```python
from build123d import *

# Parameters (mm, degrees)
SALIENTE_EXTRUIR1_DEPTH = 220
CORTAR_EXTRUIR2_DEPTH   = 14
CROQUIS2_9_W            = 24
CROQUIS2_9_H            = 1
CROQUIS2_9_W_2          = 5
CORTAR_EXTRUIR3_DEPTH   = 3
CROQUIS4_R              = 1.5
CORTAR_EXTRUIR4_DEPTH   = 10
CROQUIS5_R              = 2
CORTAR_EXTRUIR5_DEPTH   = 36
CROQUIS6_W              = 55
CROQUIS6_H              = 15
CORTAR_EXTRUIR7_DEPTH   = 10
CORTAR_EXTRUIR8_DEPTH   = 30


with BuildPart() as part:
    # Croquis1 → Saliente-Extruir1 (new body)
    with BuildSketch(Plane.XY):
        with BuildLine():
            Line((0, 37), (0, 8.15))
            ThreePointArc((0, 8.15), (-8.15, 0), (0, -8.15))
            Line((0, -8.15), (0, -37))
            Line((0, -37), (-33, -37))
            ThreePointArc((-33, -37), (-34.414213562, -36.414213562), (-35, -35))
            Line((-35, -35), (-35, 35))
            ThreePointArc((-35, 35), (-34.414213562, 36.414213562), (-33, 37))
            Line((-33, 37), (0, 37))
        make_face()
    extrude(amount=SALIENTE_EXTRUIR1_DEPTH)

    # Croquis2 → Cortar-Extruir2 (cut)
    with BuildSketch(Plane.ZY.offset(35)):
        Polygon((50.34, -1.15), (82.34, -1.15), (82.34, -17.5), (156.34, -17.5), (156.34, -1.15), (169.34, -1.15), (169.34, -13.5), (196.34, -13.5), (196.34, 13.5), (169.34, 13.5), (169.34, 1.15), (156.34, 1.15), (156.34, 17.5), (82.34, 17.5), (82.34, 1.15), (50.34, 1.15), (50.34, 10.5), (10, 10.5), (10, -10.5), (50.34, -10.5), align=None)
    extrude(amount=-CORTAR_EXTRUIR2_DEPTH, mode=Mode.SUBTRACT)

    # Croquis2_9 → Cortar-Extruir3 (cut)
    with BuildSketch(Plane.ZY.offset(35)):
        Polygon((54.34, 1.15), (54.34, 2.15), (54.34, 14.5), (6, 14.5), (6, -14.5), (54.34, -14.5), (54.34, -2.15), (54.34, -1.15), (50.34, -1.15), (50.34, -10.5), (10, -10.5), (10, 10.5), (50.34, 10.5), (50.34, 1.15), align=None)
        with Locations((66.34, 1.65)):
            Rectangle(CROQUIS2_9_W, CROQUIS2_9_H)
        with Locations((66.34, -1.65)):
            Rectangle(CROQUIS2_9_W, CROQUIS2_9_H)
        Polygon((78.34, 21.5), (78.34, 2.15), (78.34, 1.15), (82.34, 1.15), (82.34, 17.5), (156.34, 17.5), (156.34, 1.15), (160.34, 1.15), (160.34, 2.15), (160.34, 21.5), align=None)
        Polygon((82.34, -1.15), (78.34, -1.15), (78.34, -2.15), (78.34, -21.5), (160.34, -21.5), (160.34, -2.15), (160.34, -1.15), (156.34, -1.15), (156.34, -17.5), (82.34, -17.5), align=None)
        with Locations((162.84, 1.65)):
            Rectangle(CROQUIS2_9_W_2, CROQUIS2_9_H)
        with Locations((162.84, -1.65)):
            Rectangle(CROQUIS2_9_W_2, CROQUIS2_9_H)
        Polygon((165.34, 17.5), (165.34, 2.15), (165.34, 1.15), (169.34, 1.15), (169.34, 13.5), (196.34, 13.5), (196.34, -13.5), (169.34, -13.5), (169.34, -1.15), (165.34, -1.15), (165.34, -2.15), (165.34, -17.5), (200.34, -17.5), (200.34, 17.5), align=None)
    extrude(amount=-CORTAR_EXTRUIR3_DEPTH, mode=Mode.SUBTRACT)

    # Croquis4 → Cortar-Extruir4 (cut)
    with BuildSketch(Plane.ZY.offset(35)):
        with Locations((8, 12.5)):
            Circle(CROQUIS4_R)
        with Locations((8, -12.5)):
            Circle(CROQUIS4_R)
        with Locations((52.34, 12.5)):
            Circle(CROQUIS4_R)
        with Locations((52.34, -12.5)):
            Circle(CROQUIS4_R)
        with Locations((80.34, 19.5)):
            Circle(CROQUIS4_R)
        with Locations((158.34, 19.5)):
            Circle(CROQUIS4_R)
        with Locations((80.34, -19.5)):
            Circle(CROQUIS4_R)
        with Locations((158.34, -19.5)):
            Circle(CROQUIS4_R)
        with Locations((167.34, 15.5)):
            Circle(CROQUIS4_R)
        with Locations((198.34, 15.5)):
            Circle(CROQUIS4_R)
        with Locations((167.34, -15.5)):
            Circle(CROQUIS4_R)
        with Locations((198.34, -15.5)):
            Circle(CROQUIS4_R)
    extrude(amount=-CORTAR_EXTRUIR4_DEPTH, mode=Mode.SUBTRACT)

    # Croquis5 → Cortar-Extruir5 (cut, through all)
    with BuildSketch(Plane.ZY.offset(35)):
        with Locations((40, 31.5)):
            Circle(CROQUIS5_R)
        with Locations((40, -31.5)):
            Circle(CROQUIS5_R)
        with Locations((180, 31.5)):
            Circle(CROQUIS5_R)
        with Locations((180, -31.5)):
            Circle(CROQUIS5_R)
    extrude(amount=-CORTAR_EXTRUIR5_DEPTH, mode=Mode.SUBTRACT)

    # Croquis6 → Cortar-Extruir7 (cut)
    with BuildSketch(Plane.ZY.offset(21)):
        with Locations((128.84, 10)):
            Rectangle(CROQUIS6_W, CROQUIS6_H)
    extrude(amount=-CORTAR_EXTRUIR7_DEPTH, mode=Mode.SUBTRACT)

    # Croquis12 → Cortar-Extruir8 (cut)
    with BuildSketch(Plane(origin=(0, 37, 0), x_dir=(1, 0, 0), z_dir=(0, 1, 0))):
        Polygon((-19.700712137, -82.34), (-18.7, -82.34), (-18.7, -106.34), (-28.2, -106.34), (-28.2, -82.34), align=None)
    extrude(amount=-CORTAR_EXTRUIR8_DEPTH, mode=Mode.SUBTRACT)


solid = part.part
```
Read the model definition and answer for the solid it produces. Units are mm, in the model's axes. A direction names the side the tool comes from. Coordinates: 2 decimals unless noted, no trailing zeros. Order: outer loops, then holes, each group sorted by start corner. A loop starts at its lowest first (then second) coordinate and runs counter-clockwise, first axis right, second up. Notation, with made-up numbers: (-20, -28.5) - (-6, -28.5) arc R16 ccw to (-6, -21.5) - close; hole circle Ø9 at (76.25, 15.25). An arc over 180 degrees is marked (long way). Answer as a JSON object with one key per item and string values. Group by question number.
Item 1: Flat-ended cylindrical pins translate along their axes: P1, Ø10, axis at y = 12, z = 140.5, coming from the -X side; P2, Ø2, axis at y = 16, z = 79.5, coming from the -X side; P3, Ø3, axis at y = 2, z = 25.5, coming from the -X side; P4, Ø3, axis at y = 31.5, z = 180, coming from the +X side. Find the tip coordinate at first contact, or state that the pin passes through.
Item 2: Consider probe 1 along Y at (x, z) = (-17.5, 40); probe 2 along Y at (x, z) = (-28.5, 80.34); probe 3 along X at (y, z) = (18, 89). Determine where each line is inside the solid, lowest interval first. Write a range as from..to.
Item 3: Section D-D (z = 203.5) is taken. Give the vertices of the cut face in (x, y), plus the area to 3 significant figures.
Item 4: Section B-B (x = -6) is taken. Give the vertices of the cut face in (y, z), plus the area to 3 significant figures.
Item 5: A tool of negligible diameter and unlimited length cuts with its end or side. For faces 1 (the face through (-22, 17.5, 128)), 2 (the face through (-23, 27, 106.34)), 3 (the face through (-17, 1, 0)), from which of +Z, -Z, +X, -X, +Y, -Y can it reach the whole face along a straight path? Write none if from no direction.
Item 6: The mould has two halves that part along Y. Classify faces 4 (the face through (-16, -37, 108)), 5 (the face through (-18.7, 22, 94)), 6 (the face through (-17, 37, 108)), 7 (the face through (-27, -1.15, 163)): +Y half, -Y half, draft (parallel to the pull), parting line (faces both ways), or undercut.
Item 7: Section A-A (y = 23.5) is taken. Give the vertices of the cut face in (x, z), plus the area to 3 significant figures.
Item 8: Section C-C (z = 40) is taken. Give the vertices of the cut face in (x, y), plus the area to 3 significant figures.
Results are:
{
 "1": {"P1": "stops at x = -11", "P2": "stops at x = -32", "P3": "stops at x = -21", "P4": "passes through"},
 "2": {"probe 1": "y = -37..-33.5, -29.5..29.5, 33.5..37", "probe 2": "y = -37..-21, -18..-1.15, 1.15..18, 21..37", "probe 3": "x = -32..-28.2, -18.7..0"},
 "3": {"outline": "(-35, -35) arc R2 ccw to (-33, -37) - (0, -37) - (0, -8.15) arc R8.15 cw to (0, 8.15) - (0, 37) - (-33, 37) arc R2 ccw to (-35, 35) - close", "area": "2,480 mm^2"},
 "4": {"outline": "(-37, 0) - (-5.52, 0) - (-5.52, 220) - (-37, 220) - close; (5.52, 0) - (37, 0) - (37, 220) - (5.52, 220) - close; hole circle Ø4 at (-31.5, 40); hole circle Ø4 at (-31.5, 180); hole circle Ø4 at (31.5, 40); hole circle Ø4 at (31.5, 180)", "area": "13,800 mm^2"},
 "5": {"face 1": "-X", "face 2": "+Y", "face 3": "-Z, +X, -X, +Y, -Y"},
 "6": {"face 4": "-Y half", "face 5": "draft", "face 6": "+Y half", "face 7": "undercut"},
 "7": {"outline": "(-35, 0) - (0, 0) - (0, 220) - (-35, 220) - close; hole (-28.2, 82.34) - (-18.7, 82.34) - (-18.7, 106.34) - (-28.2, 106.34) - close", "area": "7,470 mm^2"},
 "8": {"outline": "(-35, -35) arc R2 ccw to (-33, -37) - (0, -37) - (0, -33.5) - (-35, -33.5) - close; (-35, -29.5) - (0, -29.5) - (0, -8.15) arc R8.15 cw to (0, 8.15) - (0, 29.5) - (-35, 29.5) - (-35, 14.5) - (-32, 14.5) - (-32, 10.5) - (-21, 10.5) - (-21, -10.5) - (-32, -10.5) - (-32, -14.5) - (-35, -14.5) - close; (-35, 33.5) - (0, 33.5) - (0, 37) - (-33, 37) arc R2 ccw to (-35, 35) - close", "area": "1,890 mm^2"}
}
